from build123d import *

# Parameters (mm, degrees)
SKETCH_1_W          = 40
SKETCH_1_H          = 20
EXTRUDE_1_DEPTH     = 40
SKETCH_2_W          = 20
SKETCH_2_H          = 2
SKETCH_2_W_2        = 7
SKETCH_2_H_2        = 3
EXTRUDE_2_DEPTH     = 6
SKETCH_3_W          = 20
SKETCH_3_H          = 2
EXTRUDE_3_DEPTH     = 6
SKETCH_4_R          = 2
CUT_EXTRUDE_2_DEPTH = 6
SKETCH_5_R          = 6.5
EXTRUDE_4_DEPTH     = 1
SKETCH_6_R          = 5.5
EXTRUDE_5_DEPTH     = 0.5
SKETCH_7_R          = 3
EXTRUDE_6_DEPTH     = 4


with BuildPart() as part:
    # 草图1 → 凸台-拉伸1 (new body)
    with BuildSketch(Plane(origin=(0, 0, 0), x_dir=(1, 0, 0), z_dir=(0, 1, 0))):
        Rectangle(SKETCH_1_W, SKETCH_1_H)
    extrude(amount=EXTRUDE_1_DEPTH)

    # 草图2 → 凸台-拉伸2 (add)
    with BuildSketch(Plane(origin=(20, 0, 0), x_dir=(0, 0, -1), z_dir=(1, 0, 0))):
        with Locations((0, 29)):
            Rectangle(SKETCH_2_W, SKETCH_2_H)
        with Locations((0, 1.5)):
            Rectangle(SKETCH_2_W_2, SKETCH_2_H_2)
    extrude(amount=EXTRUDE_2_DEPTH)

    # 草图3 → 凸台-拉伸3 (add)
    with BuildSketch(Plane.ZY.offset(20)):
        with Locations((0, 29)):
            Rectangle(SKETCH_3_W, SKETCH_3_H)
    extrude(amount=EXTRUDE_3_DEPTH)

    # 草图4 → 切除-拉伸2 (cut)
    with BuildSketch(Plane(origin=(0, 30, 0), x_dir=(1, 0, 0), z_dir=(0, 1, 0))):
        with Locations((24.1, 5)):
            Circle(SKETCH_4_R)
        with Locations((24.1, -5)):
            Circle(SKETCH_4_R)
        with Locations((-24.1, 5)):
            Circle(SKETCH_4_R)
        with Locations((-24.1, -5)):
            Circle(SKETCH_4_R)
    extrude(amount=-CUT_EXTRUDE_2_DEPTH, mode=Mode.SUBTRACT)

    # 草图5 → 凸台-拉伸4 (add)
    with BuildSketch(Plane(origin=(0, 40, 0), x_dir=(1, 0, 0), z_dir=(0, 1, 0))):
        with Locations((10, 0)):
            Circle(SKETCH_5_R)
    extrude(amount=EXTRUDE_4_DEPTH)

    # 草图6 → 凸台-拉伸5 (add)
    with BuildSketch(Plane(origin=(0, 41, 0), x_dir=(1, 0, 0), z_dir=(0, 1, 0))):
        with Locations((10, 0)):
            Circle(SKETCH_6_R)
    extrude(amount=EXTRUDE_5_DEPTH)

    # 草图7 → 凸台-拉伸6 (add)
    with BuildSketch(Plane(origin=(0, 41.5, 0), x_dir=(1, 0, 0), z_dir=(0, 1, 0))):
        with Locations((10, 0)):
            Circle(SKETCH_7_R)
    extrude(amount=EXTRUDE_6_DEPTH)


solid = part.part
Here's how the part is built. I have some questions about the finished solid (model axes, mm). A direction names the side the tool comes from. Coordinates: 2 decimals unless noted, no trailing zeros. Order: outer loops, then holes, each group sorted by start corner. A loop starts at its lowest first (then second) coordinate and runs counter-clockwise, first axis right, second up. Notation, with made-up numbers: (61, 53) -> (75, 53) arc R9 cw to (75, 57) -> close; hole circle Ø1 at (82, 62). An arc over 180 degrees is marked (long way). Answer in a Markdown table with one row per item.
(1) I want a section at C-C on z = -8.5. List the corners of the cut face in (x, y) for me, then the cut area to 3 significant figures.
Answer key:
| item | result |
|---|---|
| outline | (-26, 28) -> (-20, 28) -> (-20, 0) -> (20, 0) -> (20, 28) -> (26, 28) -> (26, 30) -> (20, 30) -> (20, 40) -> (-20, 40) -> (-20, 30) -> (-26, 30) -> close |
| area | 1,620 mm^2 |
(2) I want a section at A-A on x = 24.1. List the corners of the cut face in (y, z) for me, then the cut area to 3 significant figures.
Answer key:
| item | result |
|---|---|
| outline | (0, -3.5) -> (3, -3.5) -> (3, 3.5) -> (0, 3.5) -> close; (28, -10) -> (30, -10) -> (30, -7) -> (28, -7) -> close; (28, -3) -> (30, -3) -> (30, 3) -> (28, 3) -> close; (28, 7) -> (30, 7) -> (30, 10) -> (28, 10) -> close |
| area | 45.0 mm^2 |
(3) I want a section at D-D on x = 10. List the corners of the cut face in (y, z) for me.
Answer key:
| item | result |
|---|---|
| outline | (0, -10) -> (40, -10) -> (40, -6.5) -> (41, -6.5) -> (41, -5.5) -> (41.5, -5.5) -> (41.5, -3) -> (45.5, -3) -> (45.5, 3) -> (41.5, 3) -> (41.5, 5.5) -> (41, 5.5) -> (41, 6.5) -> (40, 6.5) -> (40, 10) -> (0, 10) -> close |
(4) Please list where these lines run through material, in increasing order: probe 1 along Z at (x, y) = (-24, 29); probe 2 along Y at (x, z) = (-21.5, 4.75); probe 3 along Y at (x, z) = (-2, 0.75).
Answer key:
| item | result |
|---|---|
| probe 1 | -10 to -7, -3 to 3, 7 to 10 |
| probe 2 | 28 to 30 |
| probe 3 | 0 to 40 |
(5) On a 3-axis mill with a long thin cutter (end or side, diameter ignored), from which of +Z, -Z, +X, -X, +Y, -Y can I reach the whole of each face in a straight line? I mean faces 5 (the face through (22.1, 29.01, 4.92)), 6 (the face through (23, 3, 0)), 7 (the face through (-20, 14, 0)). Say none if no direction works.
Answer key:
| item | result |
|---|---|
| face 5 | +Y |
| face 6 | +Z, -Z, +X |
| face 7 | +Z, -Z, -X, -Y |
(6) Thinking about a two-plate mould opening in Z: for faces 1 (the face through (-26, 29, 0)), 2 (the face through (16.2, 40.49, -1.95)), 3 (the face through (23, 1, 3.5)), 4 (the face through (-22.1, 29.01, 5.08)), which applies, +Z half, -Z half, draft (parallel to the pull), parting line (faces both ways), or undercut?
Answer key:
| item | result |
|---|---|
| face 1 | draft |
| face 2 | parting line |
| face 3 | +Z half |
| face 4 | undercut |
(7) Will these pins go through, and if not, where does the flat tip stop? pin 1 Ø1.5 at (y, z) = (6, -8) entering from +X; pin 2 Ø6 at (y, z) = (9.5, 4.5) entering from -X; pin 3 Ø10 at (y, z) = (25, -3) entering from -X; pin 4 Ø0.9 at (x, y) = (24, 1.5) entering from +Z.
Answer key:
| item | result |
|---|---|
| pin 1 | x = 20 |
| pin 2 | x = -20 |
| pin 3 | x = -26 |
| pin 4 | z = 3.5 |
(8) I want a section at B-B on x = -24.1. List the corners of the cut face in (y, z) for me.
Answer key:
| item | result |
|---|---|
| outline | (28, -10) -> (30, -10) -> (30, -7) -> (28, -7) -> close; (28, -3) -> (30, -3) -> (30, 3) -> (28, 3) -> close; (28, 7) -> (30, 7) -> (30, 10) -> (28, 10) -> close |
